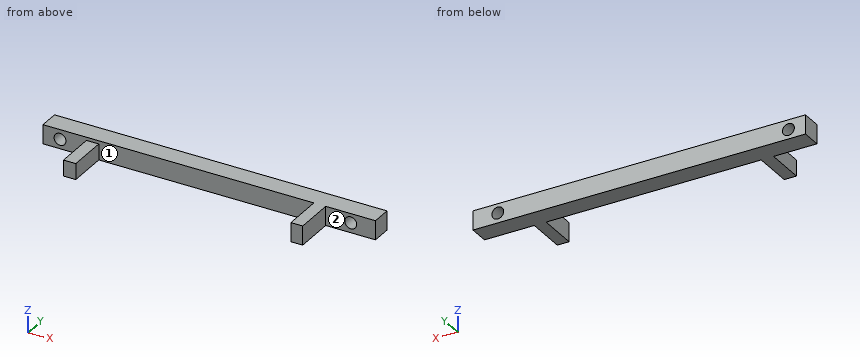
from build123d import *

# Parameters (mm, degrees)
F0_W      = 213.4951800108
F0_H      = 12.2640058398
F1_DEPTH  = 12.7
F3_D      = 7.62
F5_D      = 7.62
F6_W      = 7.8961476684
F6_H      = 5.2659846842
F7_DEPTH  = 25.4
F8_W      = 7.5909867883
F8_H      = 12.2640058398
F9_DEPTH  = 25.4
F10_W     = 7.8961476684
F10_H     = 4.9674399197
F11_DEPTH = 25.4
F12_DEPTH = 12.7


with BuildPart() as f1:
    # F0 (on Front) → F1 (new body)
    with BuildSketch(Plane.XZ):
        with Locations((31.6951796412, 41.8346524239)):
            Rectangle(F0_W, F0_H)
    extrude(amount=F1_DEPTH)

    # F3 (through all)
    with Locations(Plane.XZ.offset(12.7)):
        with Locations((-64.0981197357, 41.7276620865)):
            Hole(F3_D / 2)

    # F5 (through all)
    with Locations(Plane.XZ.offset(12.7)):
        with Locations((122.5372925401, 42.0484915376)):
            Hole(F5_D / 2)

    # F6 (on Front) → F7 (join)
    with BuildSketch(Plane.XZ):
        with Locations((-43.1862734258, 43.3030817658)):
            Rectangle(F6_W, F6_H)
    extrude(amount=F7_DEPTH)

    # F8 (on face) → F9 (join)
    with BuildSketch(Plane.XZ.offset(12.7)):
        with Locations((102.6745773852, 41.8346524239)):
            Rectangle(F8_W, F8_H)
    extrude(amount=F9_DEPTH)

    # F10 (on face) → F11 (join)
    with BuildSketch(Plane.XZ.offset(12.7)):
        with Locations((-43.1862734258, 38.1863694638)):
            Rectangle(F10_W, F10_H)
    extrude(amount=F11_DEPTH)

    # F12 (add): a face of the model
    f12_faces = [f1.faces().sort_by_distance(p)[0] for p in [
        (-43.1862734258, -25.4, 43.3030817658),
    ]]
    extrude(f12_faces, amount=F12_DEPTH)


solid = f1.part
Work out the finished part from the listing and answer in its coordinate system (mm). Face numbers are marked on the shaded views. Round coordinates to 2 decimals unless told otherwise and drop trailing zeros. Write each loop counter-clockwise with the first axis right and the second up, starting at its lowest first coordinate (ties: lowest second). Pieces come first, ordered by that corner, then holes.
1) A cutting plane is placed at A-A (y = -29.5). Give the vertices of the cut face in (x, z), plus the area to 3 significant figures.
2) Straight lines are drawn through the part: line 1 (X direction, y = -30.5, z = 44.75); line 2 (Y direction, x = -38, z = 43.5); line 3 (X direction, y = -4, z = 40.5). For each, find the intervals that lie inside material, in ascending order.
3) Given pin 1 Ø2.5 at (x, y) = (-45, -29) entering from +Z; pin 2 Ø2 at (y, z) = (-16, 42) entering from +X; pin 3 Ø3.5 at (x, z) = (127.5, 41) entering from -Y; pin 4 Ø4.5 at (x, z) = (-64.1, 41.73) entering from -Y, each flat-ended and moving along its own axis, determine where each tip first touches the part or whether it passes through.
4) A cutting plane is placed at B-B (x = 59). Give the vertices of the cut face in (y, z).
5) A cutting plane is placed at C-C (y = -2.5). Give the vertices of the cut face in (x, z), plus the area to 3 significant figures.
6) The mould has two halves that part along X. Classify the marked faces 1 and 2: pulls with the +X half, pulls with the -X half, needs draft (parallel to the pull), parting line crosses it, or undercut.
Completed:
1. outline: (-47.13, 35.7) - (-39.24, 35.7) - (-39.24, 45.94) - (-47.13, 45.94) - close; (98.88, 35.7) - (106.47, 35.7) - (106.47, 47.97) - (98.88, 47.97) - close
1. area: 174 mm2
2. line 1: x = -47.13 to -39.24, 98.88 to 106.47
2. line 2: y = -12.7 to 0
2. line 3: x = -75.05 to -67.7, -60.49 to 119.06, 126.02 to 138.44
3. pin 1: stops at z = 45.94
3. pin 2: stops at x = 106.47
3. pin 3: stops at y = -12.7
3. pin 4: passes through
4. outline: (-12.7, 35.7) - (0, 35.7) - (0, 47.97) - (-12.7, 47.97) - close
5. outline: (-75.05, 35.7) - (138.44, 35.7) - (138.44, 47.97) - (-75.05, 47.97) - close; hole circle Ø7.62 at (-64.1, 41.73); hole circle Ø7.62 at (122.54, 42.05)
5. area: 2,530 mm2
6. face 1: undercut
6. face 2: needs draft
